Autodesk Inventor part; units mm, degrees
ref_plane "YZ Plane" through (0, 0, 0) normal (1, 0, 0) x (0, 1, 0)
ref_plane "XZ Plane" through (0, 0, 0) normal (0, 1, 0) x (-1, 0, 0)
ref_plane "XY Plane" through (0, 0, 0) normal (0, 0, 1) x (1, 0, 0)
sketch "Sketch1" plane through (0, 0, 0) normal (0, 1, 0) x (-1, 0, 0)
  circle A0 centre (0, 0) radius 4.1275
  dimension "d0" = 8.255
extrude "Extrusion1" add sketch "Sketch1" along normal blind 5.08
sketch "Sketch2" plane through (0, 5.08, 0) normal (0, 1, 0) x (1, 0, 0)
  circle A0 centre (0, 0) radius 4.1275
  arc A1 (2.2225, 19.6215) -> (-2.2225, 19.6215) centre (0, 19.6215) ccw
  line L0 (-2.2225, 19.6215) -> (-4.1041, 0.4388)
  line L1 (4.1041, 0.4388) -> (2.2225, 19.6215)
  arc A2 (-4.1041, 0.4388) -> (4.1041, 0.4388) centre (0, 0) ccw
  dimension "d4" = 4.445
extrude "Extrusion2" add sketch "Sketch2" against normal blind 2.032
sketch "Sketch3" plane through (0, 5.08, 0) normal (0, 1, 0) x (1, 0, 0)
  arc A0 (2.2225, 19.6215) -> (-2.2225, 19.6215) centre (0, 19.6215) ccw
  circle A1 centre (0, 19.6215) radius 0.635
  circle A2 centre (0, 17.0815) radius 0.6558
  circle A3 centre (0, 14.5415) radius 0.6558
  circle A4 centre (0, 12.0015) radius 0.6558
  point P0 (0, 0)
  dimension "d7" = 1.27
extrude "Extrusion3" cut sketch "Sketch3" against normal blind 3.6195
properties part number "ServoHorn"
CAD build for the part. Positions are in the model's coordinates, mm. Give positions to 0.01 mm unless a question says otherwise; leave off trailing zeros. Write each loop counter-clockwise with the first axis right and the second up, starting at its lowest first coordinate (ties: lowest second). Pieces come first, ordered by that corner, then holes. Notation, with made-up numbers: (39, 59) -> (57, 59) arc R28 cw to (57, 77) -> close; hole circle Ø4 at (86.25, 59). An arc over 180 degrees is marked (long way). Write each question's results on one line, items separated by ' | '.
1. Cut at C-C, the plane x = 3.75. Write the cut outline in (y, z).
Geometry check:
outline: (0, -1.72) -> (3.05, -1.72) -> (3.05, -4.05) -> (5.08, -4.05) -> (5.08, 1.72) -> (0, 1.72) -> close
2. Wall check: probe 1 along Z at (x, y) = (0, 3.6); probe 2 along Z at (x, y) = (-0.5, 4.7); probe 3 along Y at (x, z) = (-0.25, -9.5). Give the ranges that are in metal, low to high. Write a range as [from, to].
Geometry check:
probe 1: [-21.84, -20.26], [-18.99, -17.74], [-16.43, -15.2], [-13.89, -12.66], [-11.35, 4.13] | probe 2: [-21.79, -20.01], [-19.23, -17.51], [-16.66, -14.97], [-14.12, -12.43], [-11.58, 4.1] | probe 3: [3.05, 5.08]
3. Drop flat-ended pins along their axis: P1, Ø2, axis at y = 3, z = -13.5, coming from the +X side; P2, Ø1.2, axis at x = 0, z = -12, coming from the -Y side; P3, Ø2, axis at x = -2, y = 3.5, coming from the -Z side; P4, Ø2, axis at y = 2.5, z = -19, coming from the +X side. Give the stop position or say it passes through.
Geometry check:
P1: x = 2.92 | P2: through | P3: z = -21.61 | P4: x = 2.37
4. Two-plate mould, pull along Z, no slides. Class faces 1 (the cylindrical face through (0.89, 1.94, 4.03)), 2 (the flat face through (0, 5.08, -6)), 3 (the cylindrical face through (-0.08, 4.08, -20.25)): pulls with the +Z half, pulls with the -Z half, needs draft (parallel to the pull), parting line crosses it, or undercut.
Geometry check:
face 1: parting line crosses it | face 2: needs draft | face 3: undercut
5. Cut at A-A, the plane x = 0. Write the cut outline in (y, z), then the cut area to 3 significant figures.
Geometry check:
outline: (0, -4.13) -> (3.05, -4.13) -> (3.05, -11.35) -> (5.08, -11.35) -> (5.08, 4.13) -> (0, 4.13) -> close; (3.05, -21.84) -> (5.08, -21.84) -> (5.08, -20.26) -> (3.05, -20.26) -> close; (3.05, -18.99) -> (5.08, -18.99) -> (5.08, -17.74) -> (3.05, -17.74) -> close; (3.05, -16.43) -> (5.08, -16.43) -> (5.08, -15.2) -> (3.05, -15.2) -> close; (3.05, -13.89) -> (5.08, -13.89) -> (5.08, -12.66) -> (3.05, -12.66) -> close | area: 67.4 mm²
6. Cut at D-D, the plane y = 2.25. Write the cut outline in (x, z) (1 decimal).
Geometry check:
outline: circle Ø8.3 at (0, 0)
7. Cut at B-B, the plane y = 4.1. Write the cut outline in (x, z) (1 decimal).
Geometry check:
outline: (-4.1, -0.4) -> (-2.2, -19.6) arc R2.2 ccw to (2.2, -19.6) -> (4.1, -0.4) arc R4.1 ccw (long way) to start; hole circle Ø1.3 at (0, -17.1); hole circle Ø1.3 at (0, -14.5); hole circle Ø1.3 at (0, -12); hole circle Ø1.3 at (0, -19.6)
